CAD build for the part. Positions are in the model's coordinates, mm. Face numbers are marked on the shaded views. Coordinates: 2 decimals unless noted, no trailing zeros. Loops run counter-clockwise (first coordinate to the right, second up) from the corner with the lowest first, then second, coordinate; pieces in that order, holes last. Notation, with made-up numbers: (16.5, 58) -> (68.5, 58) arc R24 cw to (68.5, 79) -> close; hole circle Ø8 at (-12, 38). An arc over 180 degrees is marked (long way). Write item = value, one per line. Start each with the question number.
(1) Pull direction X, two halves, no side cores. Call the marked faces 1, 2, 3 and 4: +X half, -X half, draft (parallel to the pull), parting line (faces both ways), or undercut.
(2) Band-saw the part on B-B (y = -6.5). Write the cut outline in (x, z).
(3) Band-saw the part on A-A (x = -80). Write the cut outline in (y, z).
(4) Drill centre lines: line 1 (Y direction, x = 23, z = 6.25); line 2 (X direction, y = 8, z = 12.25); line 3 (Z direction, x = 14, y = -1.5). Where is each one in solid material? Low to high. Write a range as from..to.
(5) Band-saw the part on C-C (z = 3.25). Write the cut outline in (x, y), and give its area (3 significant figures).
(6) Flat gauge pins, fed straight in: P1, Ø10, axis at x = 80, y = 5, coming from the -Z side; P2, Ø4, axis at x = 28.5, y = 10.5, coming from the +Z side. Where does each tip first touch, or does it go through?
(7) Band-saw the part on D-D (x = 23). Write the cut outline in (y, z).
```python
from build123d import *

# Parameters (mm, degrees)
SKETCH1_W                                           = 200
SKETCH1_H                                           = 50
EXTRUDE1_DEPTH                                      = 16
SKETCH2_W                                           = 75
SKETCH2_H                                           = 50
EXTRUDE2_DEPTH                                      = 0.5
M6_TAPPED_HOLE1_D                                   = 5
CBORE_FOR_M6_HEX_SOCKET_HEAD_CAP_SCREW1_D           = 6.6
CBORE_FOR_M6_HEX_SOCKET_HEAD_CAP_SCREW1_CBORE_D     = 11
CBORE_FOR_M6_HEX_SOCKET_HEAD_CAP_SCREW1_CBORE_DEPTH = 6.4


with BuildPart() as part:
    # Sketch1 → Extrude1 (new body)
    with BuildSketch(Plane.XY):
        Rectangle(SKETCH1_W, SKETCH1_H)
    extrude(amount=EXTRUDE1_DEPTH)

    # Sketch2 → Extrude2 (cut)
    with BuildSketch(Plane.XY.offset(16)):
        Rectangle(SKETCH2_W, SKETCH2_H)
    extrude(amount=-EXTRUDE2_DEPTH, mode=Mode.SUBTRACT)

    # M6 Tapped Hole1 (through all)
    with Locations(Plane.XY.offset(15.5)):
        with Locations((-23, 6.5), (-23, -6.5), (23, -6.5), (23, 6.5)):
            Hole(M6_TAPPED_HOLE1_D / 2)

    # CBORE for M6 Hex Socket Head Cap Screw1 (through all)
    with Locations(Plane(origin=(0, 0, 0), x_dir=(-1, 0, 0), z_dir=(0, 0, -1))):
        with Locations((-80, 5), (80, 5)):
            CounterBoreHole(CBORE_FOR_M6_HEX_SOCKET_HEAD_CAP_SCREW1_D / 2, CBORE_FOR_M6_HEX_SOCKET_HEAD_CAP_SCREW1_CBORE_D / 2, CBORE_FOR_M6_HEX_SOCKET_HEAD_CAP_SCREW1_CBORE_DEPTH)


solid = part.part
```
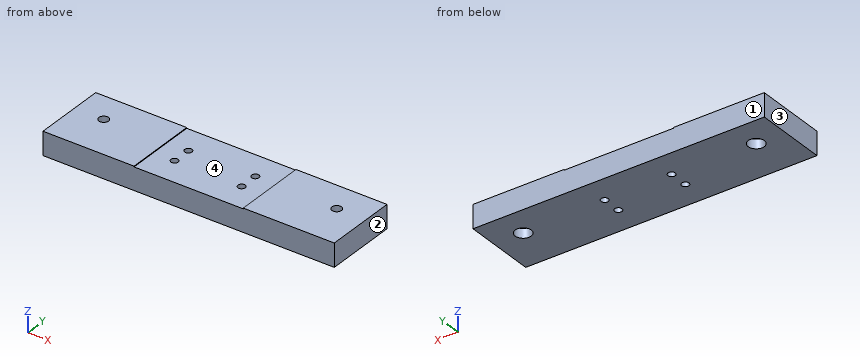
Findings below:
q1.face_1 = draft
q1.face_2 = +X half
q1.face_3 = -X half
q1.face_4 = undercut
q2.outline = (-100, 0) -> (-25.5, 0) -> (-25.5, 15.5) -> (-37.5, 15.5) -> (-37.5, 16) -> (-100, 16) -> close; (-20.5, 0) -> (20.5, 0) -> (20.5, 15.5) -> (-20.5, 15.5) -> close; (25.5, 0) -> (100, 0) -> (100, 16) -> (37.5, 16) -> (37.5, 15.5) -> (25.5, 15.5) -> close
q3.outline = (-25, 0) -> (-0.5, 0) -> (-0.5, 6.4) -> (1.7, 6.4) -> (1.7, 16) -> (-25, 16) -> close; (8.3, 6.4) -> (10.5, 6.4) -> (10.5, 0) -> (25, 0) -> (25, 16) -> (8.3, 16) -> close
q4.line_1 = -25..-9, -4..4, 9..25
q4.line_2 = -100..-81.37, -78.63..-25, -21..21, 25..78.63, 81.37..100
q4.line_3 = 0..15.5
q5.outline = (-100, -25) -> (100, -25) -> (100, 25) -> (-100, 25) -> close; hole circle Ø11 at (-80, 5); hole circle Ø5 at (-23, -6.5); hole circle Ø5 at (-23, 6.5); hole circle Ø5 at (23, -6.5); hole circle Ø5 at (23, 6.5); hole circle Ø11 at (80, 5)
q5.area = 9,730 mm²
q6.P1 = 6.4
q6.P2 = 15.5
q7.outline = (-25, 0) -> (-9, 0) -> (-9, 15.5) -> (-25, 15.5) -> close; (-4, 0) -> (4, 0) -> (4, 15.5) -> (-4, 15.5) -> close; (9, 0) -> (25, 0) -> (25, 15.5) -> (9, 15.5) -> close
